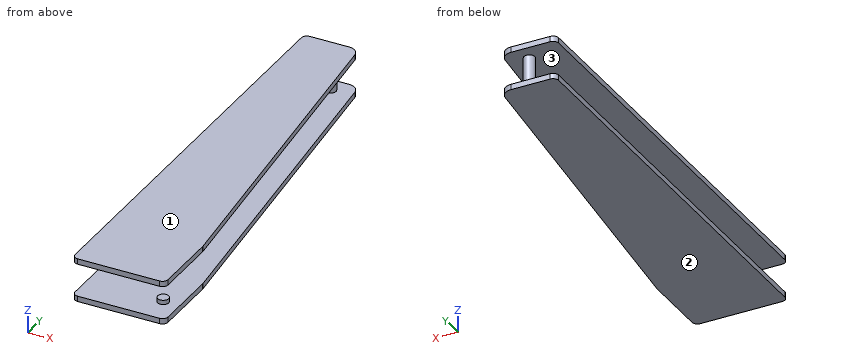
from build123d import *

# Parameters (mm, degrees)
BOSS_EXTRUDE1_DEPTH     = 5
SKETCH3_R               = 5
BOSS_EXTRUDE2_DEPTH     = 30
BOSS_EXTRUDE3_DEPTH     = 5
CUT_EXTRUDE3_DEPTH      = 11
CUT_EXTRUDE3_DEPTH_BACK = 11
SKETCH5_R               = 5


with BuildPart() as part:
    # Sketch2 → Boss-Extrude1 (new body)
    with BuildSketch(Plane.XY):
        with BuildLine():
            Line((0.936211321, 291.039120216), (34.945864928, -34.48185003))
            ThreePointArc((34.945864928, -34.48185003), (34.986457062, -35.000705547), (35, -35.520970246))
            Line((35, -35.520970246), (35, -95))
            ThreePointArc((35, -95), (33.535533906, -98.535533906), (30, -100))
            Line((30, -100), (-45, -100))
            ThreePointArc((-45, -100), (-48.535533906, -98.535533906), (-50, -95))
            Line((-50, -95), (-50, 295))
            ThreePointArc((-50, 295), (-48.535533906, 298.535533906), (-45, 300))
            Line((-45, 300), (-9.009653608, 300))
            ThreePointArc((-9.009653608, 300), (-2.316044797, 297.429374205), (0.936211321, 291.039120216))
        make_face()
    extrude(amount=BOSS_EXTRUDE1_DEPTH)

    # Sketch3 → Boss-Extrude2 (add)
    with BuildSketch(Plane.XY.offset(5)):
        with Locations(Location((-18, 285, 0), (0, 0, 180))):
            Circle(SKETCH3_R)
        with Locations(Location((20, -75, 0), (0, 0, 180))):
            Circle(SKETCH3_R)
    extrude(amount=BOSS_EXTRUDE2_DEPTH)

    # Sketch4 → Boss-Extrude3 (add)
    with BuildSketch(Plane.XY.offset(35)):
        with BuildLine():
            Line((35, -95), (35, -35.520970246))
            ThreePointArc((35, -35.520970246), (34.986457062, -35.000705547), (34.945864928, -34.48185003))
            Line((34.945864928, -34.48185003), (0.936211321, 291.039120216))
            ThreePointArc((0.936211321, 291.039120216), (-2.316044797, 297.429374205), (-9.009653608, 300))
            Line((-9.009653608, 300), (-45, 300))
            ThreePointArc((-45, 300), (-48.535533906, 298.535533906), (-50, 295))
            Line((-50, 295), (-50, -95))
            ThreePointArc((-50, -95), (-48.535533906, -98.535533906), (-45, -100))
            Line((-45, -100), (30, -100))
            ThreePointArc((30, -100), (33.535533906, -98.535533906), (35, -95))
        make_face()
    extrude(amount=BOSS_EXTRUDE3_DEPTH)

    # Sketch5 → Cut-Extrude3 (cut, two sides: drawn at the far end of the back side and taken through both)
    with BuildSketch(Plane.XY.offset(20).offset(-CUT_EXTRUDE3_DEPTH_BACK)):
        with Locations(Location((20, -75, 0), (0, 0, 180))):
            Circle(SKETCH5_R)
    extrude(amount=CUT_EXTRUDE3_DEPTH + CUT_EXTRUDE3_DEPTH_BACK, mode=Mode.SUBTRACT)


solid = part.part
Build history of the part. All positions in model axes, mm. Face numbers are marked on the shaded views. Give positions to 0.01 mm unless a question says otherwise; leave off trailing zeros. Order: outer loops, then holes, each group sorted by start corner. A loop starts at its lowest first (then second) coordinate and runs counter-clockwise, first axis right, second up. Notation, with made-up numbers: M 28.5,84.25 L 55.5,84.25 A24 cw 55.5,119.25 Z; hole C 88.5,63.25 d4. An arc over 180 degrees is marked long. Use one line per item in the form item = value.
Q1. Slice it at D-D, the plane z = 26. Write the cut outline in (x, y).
Conclusion:
outline = C -18,285 d10
Q2. Wall check: probe 1 along Z at (x, y) = (19, -80.5); probe 2 along X at (y, z) = (284.5, 31); probe 3 along Y at (x, z) = (-17.5, 26). Give the ranges that are in metal, low to high.
Conclusion:
probe_1 = 0 to 5, 35 to 40
probe_2 = -22.97 to -13.03
probe_3 = 280.03 to 289.97
Q3. Slice it at A-A, the plane x = -18. Write the cut outline in (y, z).
Conclusion:
outline = M -100,0 L 300,0 L 300,5 L 290,5 L 290,35 L 300,35 L 300,40 L -100,40 L -100,35 L 280,35 L 280,5 L -100,5 Z
Q4. Pull direction Z, two halves, no side cores. Call the marked faces 1, 2 and 3: released by +Z, released by -Z, zero draft, split by the parting line, or undercut.
Conclusion:
face_1 = released by +Z
face_2 = released by -Z
face_3 = undercut
Q5. Pin check, flat tip, straight feed: P1, Ø8, axis at x = 2.5, y = 160, coming from the -Z side. Stop position of the tip, or through.
Conclusion:
P1 = 0
Q6. Slice it at C-C, the plane x = 20. Write the cut outline in (y, z), and give its area (3 significant figures).
Conclusion:
outline = M -100,0 L 108.57,0 L 108.57,5 L -70,5 L -70,9 L -80,9 L -80,5 L -100,5 Z; M -100,35 L -80,35 L -80,31 L -70,31 L -70,35 L 108.57,35 L 108.57,40 L -100,40 Z
area = 2,170 mm2
Q7. Slice it at B-B, the plane y = 245. Write the cut outline in (x, z), and give its area (3 significant figures).
Conclusion:
outline = M -50,0 L 5.75,0 L 5.75,5 L -50,5 Z; M -50,35 L 5.75,35 L 5.75,40 L -50,40 Z
area = 557 mm2
